Drawing for the job (mm, zero at the part's lowest x, y, z). Round coordinates to 2 decimals unless told otherwise and drop trailing zeros. Loops run counter-clockwise (first coordinate to the right, second up) from the corner with the lowest first, then second, coordinate; pieces in that order, holes last. Notation, with made-up numbers: M -34,34 L -24,34 A16 ccw -24,64 Z; hole C 33,69 d8. An arc over 180 degrees is marked long. Answer in a Markdown table with one row per item.
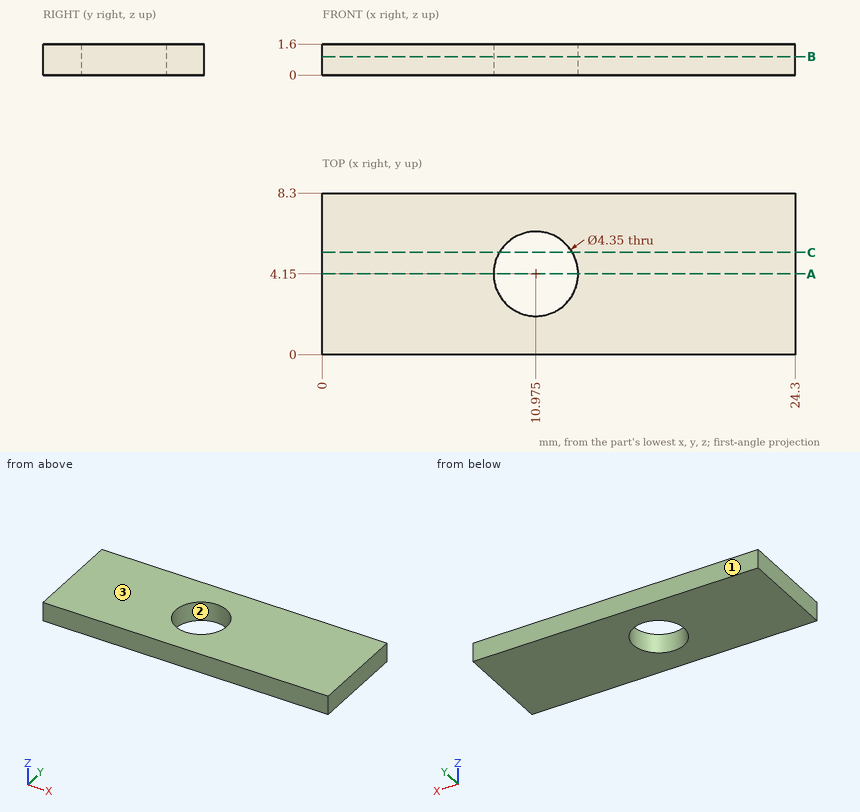
1. Saw through at A-A (y = 4.15). Write the cut outline in (x, z).
Verdict:
| item | result |
|---|---|
| outline | M 0,0 L 8.8,0 L 8.8,1.6 L 0,1.6 Z; M 13.15,0 L 24.3,0 L 24.3,1.6 L 13.15,1.6 Z |
2. Mould opens along Y. For the marked faces 1, 2 and 3 say: +Y half, -Y half, draft (parallel to the pull), parting line (faces both ways), or undercut.
Verdict:
| item | result |
|---|---|
| face 1 | +Y half |
| face 2 | undercut |
| face 3 | draft |
3. Saw through at C-C (y = 5.25). Write the cut outline in (x, z).
Verdict:
| item | result |
|---|---|
| outline | M 0,0 L 9.1,0 L 9.1,1.6 L 0,1.6 Z; M 12.85,0 L 24.3,0 L 24.3,1.6 L 12.85,1.6 Z |
4. Wall check: probe 1 along X at (y, z) = (5.75, 0.8); probe 2 along X at (y, z) = (5, 0.65); probe 3 along Y at (x, z) = (10.75, 1.3). Give the ranges that are in metal, low to high.
Verdict:
| item | result |
|---|---|
| probe 1 | x = 0 to 9.5, 12.45 to 24.3 |
| probe 2 | x = 0 to 8.97, 12.98 to 24.3 |
| probe 3 | y = 0 to 1.99, 6.31 to 8.3 |
5. Pin check, flat tip, straight feed: pin 1 (2.5 mm diameter, centred on x = 10.975, y = 4.15, fed in from +Z). Stop position of the tip, or through.
Verdict:
| item | result |
|---|---|
| pin 1 | passes through |
6. Saw through at B-B (z = 0.95). Write the cut outline in (x, y) (3 decimals).
Verdict:
| item | result |
|---|---|
| outline | M 0,0 L 24.3,0 L 24.3,8.3 L 0,8.3 Z; hole C 10.975,4.15 d4.35 |
